Check sheet for the modelled part. Datum: model origin and axes. Units: mm. A direction names the side the tool comes from. Give positions to 0.01 mm unless a question says otherwise; leave off trailing zeros. Order: outer loops, then holes, each group sorted by start corner. A loop starts at its lowest first (then second) coordinate and runs counter-clockwise, first axis right, second up.
```python
from build123d import *

# Parameters (mm, degrees)
F0_W     = 200
F0_H     = 200
F1_DEPTH = 200
F4_T     = -2.5
F5_R     = 100
F6_DEPTH = 25


# Not quite as in the source:
# - the program builds the solid bodies; features that only make, move or delete a surface that nothing else refers to are left out


with BuildPart() as f1:
    # F0 (on Front) → F1 (new body)
    with BuildSketch(Plane.XZ):
        with Locations((2.4823185522, 0)):
            Rectangle(F0_W, F0_H)
    extrude(amount=-F1_DEPTH)

    # F4
    f4_openings = [f1.faces().sort_by_distance(p)[0] for p in [
        (2.482319, 100, 100),
    ]]
    offset(amount=F4_T, openings=f4_openings)

    # F5 (on face) → F6 (join)
    with BuildSketch(Plane.XZ):
        Circle(F5_R)
    extrude(amount=F6_DEPTH)


solid = f1.part
```
(1) Cross-section at D-D on z = -74. Enter the section's corners in (x, y), then the cut area to 3 significant figures.
Response values:
outline: (-97.52, 0) - (-67.26, 0) - (-67.26, -25) - (67.26, -25) - (67.26, 0) - (102.48, 0) - (102.48, 200) - (-97.52, 200) - close; hole (-95.02, 2.5) - (99.98, 2.5) - (99.98, 197.5) - (-95.02, 197.5) - close
area: 5,340 mm2
(2) Release check for a two-part mould opening along Y. For faces 4 (the face through (100.3, 0, 0.5)), 5 (the face through (-97.518, 99, -1)), 6 (the face through (1, 2.5, 3)) record: released by +Y, released by -Y, zero draft, split by the parting line, or undercut.
Response values:
face 4: released by -Y
face 5: zero draft
face 6: undercut
(3) Cross-section at C-C on x = -21. Enter the section's corners in (y, z), then the cut area to 3 significant figures.
Response values:
outline: (-25, -97.77) - (0, -97.77) - (0, -100) - (200, -100) - (200, 100) - (197.5, 100) - (197.5, -97.5) - (2.5, -97.5) - (2.5, 100) - (0, 100) - (0, 97.77) - (-25, 97.77) - close
area: 6,380 mm2
(4) Cross-section at B-B on y = 59. Enter the section's corners in (x, z), then the cut area to 3 significant figures.
Response values:
outline: (-97.52, -100) - (102.48, -100) - (102.48, 100) - (99.98, 100) - (99.98, -97.5) - (-95.02, -97.5) - (-95.02, 100) - (-97.52, 100) - close
area: 1,490 mm2
(5) Cross-section at A-A on z = 0. Enter the section's corners in (x, y).
Response values:
outline: (-100, -25) - (100, -25) - (100, 0) - (102.48, 0) - (102.48, 200) - (-97.52, 200) - (-97.52, 0) - (-100, 0) - close; hole (-95.02, 2.5) - (99.98, 2.5) - (99.98, 197.5) - (-95.02, 197.5) - close
(6) Gauge pin test, flat ends, axial feed: pin 1 Ø10 at (x, y) = (79.5, 73) entering from +Z; pin 2 Ø2 at (y, z) = (3.5, -26.5) entering from -X. Record the tip position at first contact, or that the pin passes through.
Response values:
pin 1: stops at z = -97.5
pin 2: stops at x = -97.52
(7) Set-up check for faces 1 (the face through (99.982, 99, 0)), 2 (the face through (-74, 0, -78)), 3 (the face through (-74, 0, 79)): record each of +Z, -Z, +X, -X, +Y, -Y from which the full face is reachable in a straight line by a thin tool's end or side.
Response values:
face 1: +Z
face 2: -Z, -X, -Y
face 3: +Z, -X, -Y
(8) Material ranges on L1, parallel to Y at x = 51.5, z = -46.5; L2, parallel to Y at x = 53, z = 91; L3, parallel to X at y = 54, z = -30, recorded low to high.
Response values:
L1: y = -25 to 2.5, 197.5 to 200
L2: y = 0 to 2.5, 197.5 to 200
L3: x = -97.52 to -95.02, 99.98 to 102.48
